The model under review builds one solid part; all positions refer to its coordinate system, in mm. A direction names the side the tool comes from. Round coordinates to 2 decimals unless told otherwise and drop trailing zeros. Order: outer loops, then holes, each group sorted by start corner. A loop starts at its lowest first (then second) coordinate and runs counter-clockwise, first axis right, second up. Notation, with made-up numbers: (-21.5, 74) -> (-8.5, 74) arc R13 cw to (-8.5, 84) -> close; hole circle Ø8 at (50.5, 13). An arc over 180 degrees is marked (long way). Use a Markdown table: item, result. Add a question column.
```python
from build123d import *

# Parameters (mm, degrees)
BOSS_EXTRUDE1_DEPTH = 1.5
BOSS_EXTRUDE5_DEPTH = 10
SKETCH2_W           = 2.8
SKETCH2_H           = 2.8
BOSS_EXTRUDE2_DEPTH = 10
SKETCH4_W           = 6
SKETCH4_H           = 6
CUT_EXTRUDE1_DEPTH  = 12.5
BOSS_EXTRUDE6_DEPTH = 11.5
SKETCH8_W           = 6
SKETCH8_H           = 6
CUT_EXTRUDE3_DEPTH  = 12.5
BOSS_EXTRUDE8_DEPTH = 10


with BuildPart() as part:
    # Sketch1 → Boss-Extrude1 (new body)
    with BuildSketch(Plane(origin=(0, 0, 0), x_dir=(1, 0, 0), z_dir=(0, 1, 0))):
        Polygon((-3, 3), (-3, 9), (3, 9), (3, 3), (9, 3), (9, -3), (3, -3), (3, -9), (-3, -9), (-3, -3), (-9, -3), (-9, 3), align=None)
    extrude(amount=BOSS_EXTRUDE1_DEPTH)

    # Sketch3 → Boss-Extrude5 (add)
    with BuildSketch(Plane(origin=(0, 1.5, 0), x_dir=(1, 0, 0), z_dir=(0, 1, 0))):
        Polygon((-3, 3), (-9, 3), (-9, -3), (-3, -3), (-3, -9), (3, -9), (3, -3), (9, -3), (9, 3), (3, 3), (3, 9), (-3, 9), align=None)
        Polygon((-1.7, 1.7), (-7.6, 1.7), (-7.6, -1.7), (-1.7, -1.7), (-1.7, -7.6), (1.7, -7.6), (1.7, -1.7), (7.6, -1.7), (7.6, 1.7), (1.7, 1.7), (1.7, 7.6), (-1.7, 7.6), align=None, mode=Mode.SUBTRACT)
    extrude(amount=BOSS_EXTRUDE5_DEPTH)

    # Sketch2 → Boss-Extrude2 (add)
    with BuildSketch(Plane(origin=(0, 1.5, 0), x_dir=(1, 0, 0), z_dir=(0, 1, 0))):
        Rectangle(SKETCH2_W, SKETCH2_H)
    extrude(amount=BOSS_EXTRUDE2_DEPTH)

    # Sketch4 → Cut-Extrude1 (cut, through all)
    with BuildSketch(Plane(origin=(0, 11.5, 0), x_dir=(1, 0, 0), z_dir=(0, 1, 0))):
        with Locations((-6, 0)):
            Rectangle(SKETCH4_W, SKETCH4_H)
    extrude(amount=-CUT_EXTRUDE1_DEPTH, mode=Mode.SUBTRACT)

    # Sketch5 → Boss-Extrude6 (add)
    with BuildSketch(Plane(origin=(0, 11.5, 0), x_dir=(1, 0, 0), z_dir=(0, 1, 0))):
        Polygon((-3, 1.7), (-1.7, 1.7), (-1.7, 1.4), (-1.4, 1.4), (-1.4, -1.4), (-1.7, -1.4), (-1.7, -1.7), (-3, -1.7), align=None)
    extrude(amount=-BOSS_EXTRUDE6_DEPTH)

    # Sketch8 → Cut-Extrude3 (cut, through all)
    with BuildSketch(Plane(origin=(0, 11.5, 0), x_dir=(1, 0, 0), z_dir=(0, 1, 0))):
        with Locations((6, 0)):
            Rectangle(SKETCH8_W, SKETCH8_H)
    extrude(amount=-CUT_EXTRUDE3_DEPTH, mode=Mode.SUBTRACT)

    # Sketch9 → Boss-Extrude8 (add)
    with BuildSketch(Plane(origin=(0, 11.5, 0), x_dir=(1, 0, 0), z_dir=(0, 1, 0))):
        Polygon((1.4, -1.4), (1.4, 1.4), (1.7, 1.4), (1.7, 1.7), (3, 1.7), (3, -1.7), (1.7, -1.7), (1.7, -1.4), align=None)
    extrude(amount=-BOSS_EXTRUDE8_DEPTH)


solid = part.part
```
Q1. Draft analysis for pull direction Z (two halves, no side actions). For faces 1 (the face through (0, 6, -7.6)), 2 (the face through (0, 6, 9)), 3 (the face through (0, 6, -9)), state which applies: released by +Z, released by -Z, zero draft, split by the parting line, or undercut.
Q2. Add section B-B, the plane y = 8.5. Give the boundary of the cut face in (x, z).
Q3. For pin 1 (1.7 mm diameter, centred on x = 0.5, z = -4.5, fed in from +Y); pin 2 (3 mm diameter, centred on x = 1.5, z = -4, fed in from +Y), all flat-tipped, find the tip position at first contact; note any pin that passes through.
Q4. For faces 4 (the face through (-3, 6, 0)), 5 (the face through (0, 1.5, -5)), list the 3-axis set-ups (+Z, -Z, +X, -X, +Y, -Y) from which the entire face can be reached by the end or side of a thin tool; tool diameter is ignored.
Q5. To check wall thickness, follow line 1 along Z through (x, y) = (1.2, 4.5); line 2 along X through (y, z) = (8.5, -4.5); line 3 along Y through (x, z) = (-0.45, 4.5). State the ranges of each line that lie inside material, in increasing order.
Q6. Add section A-A, the plane x = 1.5. Give the boundary of the cut face in (y, z).
Q7. Add section C-C, the plane z = -5. Give the boundary of the cut face in (x, y).
Return value:
| question | item | result |
|---|---|---|
| 1 | face 1 | undercut |
| 1 | face 2 | released by +Z |
| 1 | face 3 | released by -Z |
| 2 | outline | (-3, -9) -> (3, -9) -> (3, 9) -> (-3, 9) -> close; hole (-1.7, -7.6) -> (1.7, -7.6) -> (1.7, -1.4) -> (-1.7, -1.4) -> close; hole (-1.7, 1.4) -> (1.7, 1.4) -> (1.7, 7.6) -> (-1.7, 7.6) -> close |
| 3 | pin 1 | y = 1.5 |
| 3 | pin 2 | y = 11.5 |
| 4 | face 4 | +Z, -Z, -X, +Y, -Y |
| 4 | face 5 | +Y |
| 5 | line 1 | -9 to -7.6, -1.4 to 1.4, 7.6 to 9 |
| 5 | line 2 | -3 to -1.7, 1.7 to 3 |
| 5 | line 3 | 0 to 1.5 |
| 6 | outline | (0, -9) -> (11.5, -9) -> (11.5, -7.6) -> (1.5, -7.6) -> (1.5, -1.4) -> (11.5, -1.4) -> (11.5, 1.4) -> (1.5, 1.4) -> (1.5, 7.6) -> (11.5, 7.6) -> (11.5, 9) -> (0, 9) -> close |
| 7 | outline | (-3, 0) -> (3, 0) -> (3, 11.5) -> (1.7, 11.5) -> (1.7, 1.5) -> (-1.7, 1.5) -> (-1.7, 11.5) -> (-3, 11.5) -> close |
